```python
from build123d import *

# Parameters (mm, degrees)
F0_W           = 152.4
F0_H           = 63.5
F1_DEPTH       = 9.525
F2_R           = 4.365625
F3_DEPTH       = 25.4
F4_D           = 8.73125
F4_CSINK_D     = 16.66875
F4_CSINK_ANGLE = 90


# Not quite as in the source:
# - a length typed as a fraction of an inch, garbled in the dataset ("3 / 203.2 mm" for 3/8 in), is restored


with BuildPart() as f1:
    # F0 (on Front) → F1 (new body)
    with BuildSketch(Plane.XZ):
        with Locations((-2.7878060937, -27.0196995885)):
            Rectangle(F0_W, F0_H)
    extrude(amount=F1_DEPTH)

    # F2 (on face) → F3 (cut)
    with BuildSketch(Plane.XZ.offset(9.525)):
        with Locations((52.9022132752, -34.9571995885)):
            Circle(F2_R)
        with Locations((-58.2227867248, -34.9571995885)):
            Circle(F2_R)
    extrude(amount=-F3_DEPTH, mode=Mode.SUBTRACT)

    # F4 (through all)
    with Locations(Plane.XZ.offset(9.525)):
        with Locations((52.9022132752, -34.9571995885), (-58.2227867248, -34.9571995885)):
            CounterSinkHole(F4_D / 2, F4_CSINK_D / 2, counter_sink_angle=F4_CSINK_ANGLE)


solid = f1.part
```
The listing builds one solid part. Answer for the finished solid, in the listing's coordinates (mm). Give positions to 0.01 mm unless a question says otherwise; leave off trailing zeros. Write each loop counter-clockwise with the first axis right and the second up, starting at its lowest first coordinate (ties: lowest second). Pieces come first, ordered by that corner, then holes. Notation, with made-up numbers: (-32.5, 1) -> (-16.5, 1) arc R14 cw to (-16.5, 8) -> close; hole circle Ø9 at (-36.5, 81). An arc over 180 degrees is marked (long way). Write item = value, one per line. Start each with the question number.
1) The part is cut by section A-A, the plane y = -7.75. Determine the outline of the cut face in (x, z).
2) Determine the mould class of faces 1 (the face through (57.46, -5.75, -34.76)), 2 (the face through (-4, -9.525, -27)), 3 (the face through (-78.988, -5, -27)) for opening direction X: +X half, -X half, draft (parallel to the pull), parting line (faces both ways), or undercut.
3) Straight lines are drawn through the part: line 1 along X through (y, z) = (-8, -29); line 2 along X through (y, z) = (-6.25, -37); line 3 along Z through (x, y) = (48.5, -8.5). For each, find the intervals that lie inside material, in ascending order.
4) Each of these flat-tipped pins is pushed along its axis until it touches: pin 1 (1 mm diameter, centred on x = 38, z = -43, fed in from +Y); pin 2 (8 mm diameter, centred on x = 52.9, z = -34.96, fed in from +Y) (1 decimal). Where does it stop, or does it pass through?
Solutions:
q1.outline = (-78.99, -58.77) -> (73.41, -58.77) -> (73.41, 4.73) -> (-78.99, 4.73) -> close; hole circle Ø13.12 at (-58.22, -34.96); hole circle Ø13.12 at (52.9, -34.96)
q2.face_1 = undercut
q2.face_2 = draft
q2.face_3 = -X half
q3.line_1 = -78.99 to -61.52, -54.92 to 49.6, 56.2 to 73.41
q3.line_2 = -78.99 to -62.85, -53.59 to 48.27, 57.53 to 73.41
q3.line_3 = -58.77 to -40.79, -29.12 to 4.73
q4.pin_1 = 0
q4.pin_2 = through
